Input: part model. Units: mm. Frame: model coordinates. Face numbers are marked on the shaded views. A direction names the side the tool comes from. Coordinates: 2 decimals unless noted, no trailing zeros. Loops run counter-clockwise (first coordinate to the right, second up) from the corner with the lowest first, then second, coordinate; pieces in that order, holes last. Notation, with made-up numbers: M 76.5,31 L 132.5,31 A24 ccw 132.5,57 Z; hole C 52,-2.75 d4. An arc over 180 degrees is marked long. Use a Markdown table: item, result. Add a question column.
1. Draft query along X for the marked faces 3, 4 and 5. Return one class per face: +X half, -X half, draft (parallel to the pull), parting line (faces both ways), or undercut.
2. Section D-D on y = 13. Output: boundary loops of the cut face in (x, z).
3. Line query: L1, parallel to Y at x = 0, z = 1.5; L2, parallel to Y at x = 3, z = -6.5; L3, parallel to Y at x = 6.25, z = -1.75. Output: solid intervals per line, ascending. Write a range as [from, to].
4. Section A-A on x = 0. Output: boundary loops of the cut face in (y, z), then the cut area to 3 significant figures.
5. Section B-B on y = -17.5. Output: boundary loops of the cut face in (x, z).
6. Section C-C on x = 10. Output: boundary loops of the cut face in (y, z).
7. Set-up query: the marked faces 1 and 2. Return all of +Z, -Z, +X, -X, +Y, -Y with unobstructed straight access to the full face (end or side cutting, diameter ignored); none if empty.
8. Pin query (flat end, axial travel): pin 1 (1 mm diameter, centred on y = -11.5, z = -4.5, fed in from -X); pin 2 (8 mm diameter, centred on y = -2.5, z = 9, fed in from -X); pin 3 (4 mm diameter, centred on x = 9, z = 9.5, fed in from +Y); pin 4 (1.5 mm diameter, centred on x = 6, y = -13.5, fed in from +Z). Return the tip coordinate at first contact, or that it passes through.
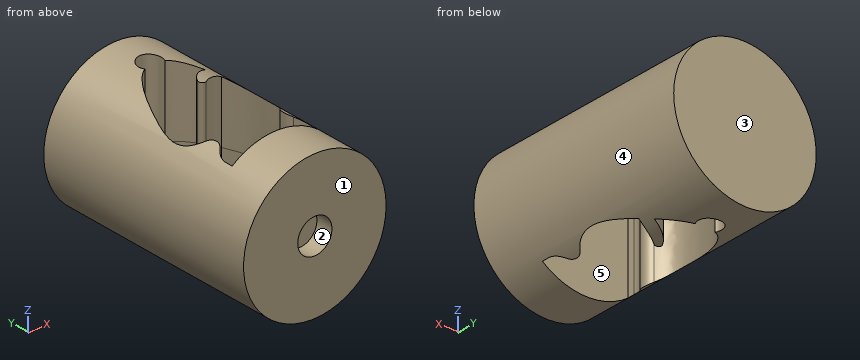
```python
from build123d import *

# Parameters (mm, degrees)
SKETCH2_R               = 12.5
BOSS_EXTRUDE1_DEPTH     = 20
CUT_EXTRUDE1_DEPTH      = 13.5
CUT_EXTRUDE1_DEPTH_BACK = 13.5
SKETCH4_R               = 3
CUT_EXTRUDE2_DEPTH      = 3


with BuildPart() as part:
    # Sketch2 → Boss-Extrude1 (new body, symmetric)
    with BuildSketch(Plane(origin=(0, 0, 0), x_dir=(1, 0, 0), z_dir=(0, 1, 0))):
        Circle(SKETCH2_R)
    extrude(amount=BOSS_EXTRUDE1_DEPTH, both=True)

    # Sketch3 → Cut-Extrude1 (cut, two sides)
    with BuildSketch(Plane.XY) as cut_extrude1_sk:
        with BuildLine():
            Line((-7.5, -12), (7.5, -12))
            Line((7.5, -12), (7.5, -10.75))
            ThreePointArc((7.5, -10.75), (7.229985685, -9.458141194), (6.465151267, -8.38257845))
            ThreePointArc((6.465151267, -8.38257845), (5.860943971, -6.976529652), (6.5, -5.585973264))
            add(Edge.make_bspline(
                [(6.399106832, 6.007513462), (6.674880251, 5.37945403), (8.419258071, 0.928997207), (8.866568078, -3.503239262), (6.5, -5.585973264)],
                knots=[0.721905241, 0.721905241, 0.721905241, 0.721905241, 0.762107282, 1, 1, 1, 1], degree=3))
            ThreePointArc((6.399106832, 6.007513462), (4.161846652, 5.358127462), (2.124976719, 4.227554084))
            ThreePointArc((2.124976719, 4.227554084), (1.410783073, 4.270418303), (1.30152237, 4.977505287))
            ThreePointArc((1.30152237, 4.977505287), (3.037185837, 6.920492718), (5.400514483, 8.017035255))
            add(Edge.make_bspline(
                [(1.754727772, 12.040348789), (3.097405823, 11.396858203), (4.352310199, 9.878271217), (5.400514483, 8.017035255)],
                knots=[0.547214619, 0.547214619, 0.547214619, 0.547214619, 0.67737121, 0.67737121, 0.67737121, 0.67737121], degree=3))
            ThreePointArc((1.754727772, 12.040348789), (0, 15), (-1.754727772, 12.040348789))
            add(Edge.make_bspline(
                [(-6.5, -5.585973264), (-9.280086296, -3.139316304), (-7.648890565, 3.398221212), (-3.956299658, 10.941083142), (-1.754727772, 12.040348789)],
                knots=[0, 0, 0, 0, 0.237892718, 0.453262832, 0.453262832, 0.453262832, 0.453262832], degree=3))
            ThreePointArc((-6.5, -5.585973264), (-5.860943971, -6.976529652), (-6.465151267, -8.38257845))
            ThreePointArc((-6.465151267, -8.38257845), (-7.229985685, -9.458141194), (-7.5, -10.75))
            Line((-7.5, -10.75), (-7.5, -12))
        make_face()
    extrude(amount=CUT_EXTRUDE1_DEPTH, mode=Mode.SUBTRACT)
    extrude(cut_extrude1_sk.sketch, amount=-CUT_EXTRUDE1_DEPTH_BACK, mode=Mode.SUBTRACT)

    # Sketch4 → Cut-Extrude2 (cut)
    with BuildSketch(Plane(origin=(0, -20, 0), x_dir=(-1, 0, 0), z_dir=(0, -1, 0))):
        Circle(SKETCH4_R)
    extrude(amount=-CUT_EXTRUDE2_DEPTH, mode=Mode.SUBTRACT)


solid = part.part
```
Answers below:
| question | item | result |
|---|---|---|
| 1 | face 3 | draft |
| 1 | face 4 | parting line |
| 1 | face 5 | undercut |
| 2 | outline | M -2,-12.34 L -2,12.34 A12.5 ccw Z; M 2,-12.34 A12.5 ccw 2,12.34 Z |
| 3 | L1 | y = [-17, -12], [15, 20] |
| 3 | L2 | y = [-20, -12], [4.79, 6.89], [11.18, 20] |
| 3 | L3 | y = [-20, -12], [-8.15, -5.85], [5.98, 20] |
| 4 | outline | M -20,-12.5 L -12,-12.5 L -12,12.5 L -20,12.5 L -20,3 L -17,3 L -17,-3 L -20,-3 Z; M 15,-12.5 L 20,-12.5 L 20,12.5 L 15,12.5 Z |
| 4 | area | 307 mm² |
| 5 | outline | C 0,0 d25; hole C 0,0 d6 |
| 6 | outline | M -20,-7.5 L 20,-7.5 L 20,7.5 L -20,7.5 Z |
| 7 | face 1 | +Z, -Z, +X, -X, -Y |
| 7 | face 2 | -Y |
| 8 | pin 1 | stops at x = -11.84 |
| 8 | pin 2 | stops at x = -11.46 |
| 8 | pin 3 | stops at y = 20 |
| 8 | pin 4 | stops at z = 11.34 |
